Autodesk Inventor part; units mm, degrees
ref_plane "YZ Plane" through (0, 0, 0) normal (1, 0, 0) x (0, 1, 0)
ref_plane "XZ Plane" through (0, 0, 0) normal (0, 1, 0) x (-1, 0, 0)
ref_plane "XY Plane" through (0, 0, 0) normal (0, 0, 1) x (1, 0, 0)
sketch "Sketch1" plane through (0, 0, 0) normal (0, 0, 1) x (1, 0, 0)
  line L0 (-5.7, -11.75) -> (5.7, -11.75)
  line L1 (5.7, -11.75) -> (5.7, 11.75)
  line L2 (5.7, 11.75) -> (-5.7, 11.75)
  line L3 (-5.7, 11.75) -> (-5.7, -11.75)
  line L4 (-5.7, -11.75) -> (5.7, 11.75) construction
  line L5 (5.7, -11.75) -> (-5.7, 11.75) construction
  line L6 (5.7, 11.75) -> (-5.7, 11.75)
  line L7 (-5.7, 11.75) -> (-5.7, 16.15)
  line L8 (-5.7, 16.15) -> (5.7, 16.15)
  line L9 (5.7, 16.15) -> (5.7, 11.75)
  circle A0 centre (-2.7, 14.15) radius 1.3
  circle A1 centre (2.7, 14.15) radius 1.3
  circle A2 centre (-2.7, -14.15) radius 1.3
  circle A3 centre (2.7, -14.15) radius 1.3
  line L10 (-5.7, -11.75) -> (5.7, -11.75)
  line L11 (5.7, -11.75) -> (5.7, -16.15)
  line L12 (5.7, -16.15) -> (-5.7, -16.15)
  line L13 (-5.7, -16.15) -> (-5.7, -11.75)
  point P0 (0, 0)
  dimension "d0" = 11.4
  dimension "d1" = 23.5
  dimension "d2" = 4.4
  dimension "d3" = 2.6
  dimension "d4" = 3
  dimension "d5" = 2.4
  dimension "d6" = 4.4
  dimension "d7" = 3
  dimension "d8" = 3
  dimension "d9" = 3
  dimension "d10" = 2.4
  dimension "d11" = 2.4
  dimension "d18" = 2.4
extrude "Extrusion1" add sketch "Sketch1" along normal blind 8 and the other way blind 20 contours L3 L2 L1 L0
extrude "Extrusion2" add sketch "Sketch1" along normal blind 2 contours L7 L8 L9 L2
extrude "Extrusion3" add sketch "Sketch1" along normal blind 2 contours L0 L11 L12 L13
sketch "Sketch2" plane through (0, 0, 8) normal (0, 0, 1) x (1, 0, 0)
  line L0 (5.7, -11.75) -> (5.7, 11.75)
  circle A0 centre (-0.015, 6.5) radius 1.5
  point P0 (0, 0)
  dimension "d37" = 3
  dimension "d38" = 5.715
  dimension "d39" = 6.5
extrude "Extrusion4" add sketch "Sketch2" along normal blind 4.5
equation "\"d0\" = ServoCoreWidth"
equation "\"d1\" = ServoCoreLength"
equation "\"d2\" = ServoFixationLength"
equation "\"d4\" = ServoEdgeToFixation"
equation "\"d5\" = ServoCoreToFixation"
equation "\"d6\" = ServoFixationLength"
equation "\"d7\" = ServoEdgeToFixation"
equation "\"d8\" = ServoEdgeToFixation"
equation "\"d9\" = ServoEdgeToFixation"
equation "\"d10\" = ServoCoreToFixation"
equation "\"d11\" = ServoCoreToFixation"
equation "\"d18\" = ServoCoreToFixation"
equation "\"ServoCoreToFixation\" = 2.4"
equation "\"ServoEdgeToFixation\" = 3"
equation "\"ServoCoreWidth\" = 11.4"
equation "\"ServoSpacing\" = 0.2"
equation "\"ServoCoreLength\" = 23.5"
equation "\"ServoFixationLength\" = 4.4"
equation "\"ServoScrewDiameter\" = 2"
equation "\"ServoHeadScrewTrace\" = 4.5"
equation "\"ServoHeadScrewThickness\" = 2.5"
equation "\"ServoExtendedSpacing\" = 1"
equation "\"ServoAxisToCenter\" = 6.5"
properties part number "SimplifiedServo"
Here's how the part is built. I have some questions about the finished solid (model axes, mm). A direction names the side the tool comes from. Give positions to 0.01 mm unless a question says otherwise; leave off trailing zeros. Write each loop counter-clockwise with the first axis right and the second up, starting at its lowest first coordinate (ties: lowest second). Pieces come first, ordered by that corner, then holes. Notation, with made-up numbers: M 33,84.5 L 81,84.5 A20 ccw 81,118.5 Z; hole C 24.5,-27.75 d4. An arc over 180 degrees is marked long. Put each result on its own line as item: value. Start each with the question number.
Item 1: If we section it at D-D, the plane y = 6.5: Write out the boundary of the cut face in (x, z) (3 decimals), then the cut area to 3 significant figures.
Item 2: On a 3-axis mill with a long thin cutter (end or side, diameter ignored), from which of +Z, -Z, +X, -X, +Y, -Y can I reach the whole of each face in a straight line? I mean faces 4 (the flat face through (0, 14, 0)), 5 (the cylindrical face through (0, 8, 10)), 6 (the flat face through (0, 11.75, 5)). Say none if no direction works.
Item 3: Will these pins go through, and if not, where does the flat tip stop? pin 1 (3 mm diameter, centred on x = 2.7, y = -14.15, fed in from +Z); pin 2 (3.5 mm diameter, centred on x = 2, y = 14, fed in from -Z); pin 3 (1.8 mm diameter, centred on x = -1, z = 5, fed in from -Y).
Item 4: If we section it at A-A, the plane x = 2.7: Write out the boundary of the cut face in (y, z), then the cut area to 3 significant figures.
Item 5: I need wall thicknesses on L1, parallel to Y at x = 2.7, z = 1.45; L2, parallel to X at y = -14, z = 1; L3, parallel to Z at x = 0, y = -7.5. Which ranges of each line are inside material? Lowest first, please. Write a range as from..to.
Item 6: If we section it at B-B, the plane y = 14.15: Write out the boundary of the cut face in (x, z), then the cut area to 3 significant figures.
Item 7: If we section it at C-C, the plane x = 4.75: Write out the boundary of the cut face in (y, z), then the cut area to 3 significant figures.
Item 8: Thinking about a two-plate mould opening in Y: for faces 1 (the flat face through (0, 7, 12.5)), 2 (the cylindrical face through (-1.5, 14.65, 0.99)), 3 (the flat face through (0, -11.75, 5)), which applies, +Y half, -Y half, draft (parallel to the pull), parting line (faces both ways), or undercut?
Values:
1. outline: M -5.7,-20 L 5.7,-20 L 5.7,8 L 1.485,8 L 1.485,12.5 L -1.515,12.5 L -1.515,8 L -5.7,8 Z
1. area: 333 mm²
2. face 4: -Z, +X, -X, +Y
2. face 5: +Z
2. face 6: +Z, +X, -X, +Y
3. pin 1: z = 2
3. pin 2: z = 0
3. pin 3: y = -11.75
4. outline: M -16.15,0 L -15.45,0 L -15.45,2 L -16.15,2 Z; M -12.85,0 L -11.75,0 L -11.75,-20 L 11.75,-20 L 11.75,0 L 12.85,0 L 12.85,2 L 11.75,2 L 11.75,8 L -11.75,8 L -11.75,2 L -12.85,2 Z; M 15.45,0 L 16.15,0 L 16.15,2 L 15.45,2 Z
4. area: 665 mm²
5. L1: -16.15..-15.45, -12.85..12.85, 15.45..16.15
5. L2: -5.7..-3.99, -1.41..1.41, 3.99..5.7
5. L3: -20..8
6. outline: M -5.7,0 L -4,0 L -4,2 L -5.7,2 Z; M -1.4,0 L 1.4,0 L 1.4,2 L -1.4,2 Z; M 4,0 L 5.7,0 L 5.7,2 L 4,2 Z
6. area: 12.4 mm²
7. outline: M -16.15,0 L -11.75,0 L -11.75,-20 L 11.75,-20 L 11.75,0 L 16.15,0 L 16.15,2 L 11.75,2 L 11.75,8 L -11.75,8 L -11.75,2 L -16.15,2 Z
7. area: 676 mm²
8. face 1: draft
8. face 2: undercut
8. face 3: -Y half
